Here's how the part is built. I have some questions about the finished solid (model axes, mm). A direction names the side the tool comes from. Give positions to 0.01 mm unless a question says otherwise; leave off trailing zeros. Loops run counter-clockwise (first coordinate to the right, second up) from the corner with the lowest first, then second, coordinate; pieces in that order, holes last.
Q1. Suppose I cut it at D-D (z = -16). List the corners of the cut face in (x, y) for me, and give its area (3 significant figures).
Q2. I need wall thicknesses on probe 1 along Z at (x, y) = (-2, 21); probe 2 along X at (y, z) = (17.75, -11.5); probe 3 along X at (y, z) = (29.2, -11.5) (3 decimals). Which ranges of each line are inside material? Lowest first, please.
Q3. Thinking about a two-plate mould opening in Y: for faces 1 (the face through (0, 30, -11)), 2 (the face through (2, 17, -20)), 3 (the face through (-2.5, 19, -1)), 4 (the face through (4.866, 28.521, -7.63)), which applies, pulls with the +Y half, pulls with the -Y half, needs draft (parallel to the pull), parting line crosses it, or undercut?
Q4. Suppose I cut it at B-B (z = -3.5). List the corners of the cut face in (x, y) for me (3 decimals), and give its area (3 significant figures).
Q5. Suppose I cut it at A-A (x = 2.5). Count the separate pieces of the cut face and the enclosed holes in it, and give its area (3 significant figures).
Q6. For faces 5 (the face through (3, 12, -1)), 6 (the face through (6, 15, -10)), 7 (the face through (4.55, 28.52, -4.24)), 8 (the face through (2, 1, -19)), 9 (the face through (-4, 10, -1)), which set-ups out of +Z, -Z, +X, -X, +Y, -Y let a thin tool reach every point of the face, with its end or its side?
```python
from build123d import *

# Parameters (mm, degrees)
EXTRUDE_1_DEPTH                  = 30
SKETCH_2_W                       = 4.5
SKETCH_2_H                       = 17
SKETCH_2_R                       = 1
EXTRUDE_2_DEPTH                  = 3
EXTRUDE_3_DEPTH                  = 27
PATTERN_LINEAR_1_COUNT           = 2
PATTERN_LINEAR_1_PITCH           = 5.5
PATTERN_LINEAR_2_COUNT           = 2
PATTERN_LINEAR_2_PITCH           = 5.5
CUT_EXTRUDE_1_REACH              = 39.108
SKETCH_5_W                       = 2.5
SKETCH_5_H                       = 3
PATTERN_LINEAR_3_COUNT           = 3
PATTERN_LINEAR_3_PITCH           = 7
PATTERN_LINEAR_4_COUNT           = 2
PATTERN_LINEAR_4_PITCH           = 5.5
PATTERN_LINEAR_4_COPY_1_REACH    = 39.108
PATTERN_LINEAR_4_COPY_1_SKETCH_W = 2.5
PATTERN_LINEAR_4_COPY_1_SKETCH_H = 3
PATTERN_LINEAR_4_COPY_2_REACH    = 39.108
PATTERN_LINEAR_4_COPY_2_SKETCH_W = 2.5
PATTERN_LINEAR_4_COPY_2_SKETCH_H = 3
CUT_EXTRUDE_2_REACH              = 39.108
SKETCH_6_W                       = 2.5
SKETCH_6_H                       = 5
PATTERN_LINEAR_5_COUNT           = 3
PATTERN_LINEAR_5_PITCH           = 7
PATTERN_LINEAR_7_COUNT           = 2
PATTERN_LINEAR_7_PITCH           = 5.5
PATTERN_LINEAR_7_COPY_1_REACH    = 39.108
PATTERN_LINEAR_7_COPY_1_SKETCH_W = 2.5
PATTERN_LINEAR_7_COPY_1_SKETCH_H = 5
PATTERN_LINEAR_7_COPY_2_REACH    = 39.108
PATTERN_LINEAR_7_COPY_2_SKETCH_W = 2.5
PATTERN_LINEAR_7_COPY_2_SKETCH_H = 5


with BuildPart() as part:
    # Эскиз1 → Бобышка-Вытянуть1 (new body)
    with BuildSketch(Plane(origin=(0, 0, 0), x_dir=(1, 0, 0), z_dir=(0, 1, 0))):
        Polygon((5, 0), (-5, 0), (-6, 1), (-6, 10.5), (-5, 10.5), (-5, 2), (-0.5, 2), (-0.5, 10.5), (0.5, 10.5), (0.5, 2), (5, 2), (5, 10.5), (6, 10.5), (6, 1), align=None)
    extrude_1 = extrude(amount=EXTRUDE_1_DEPTH)

    # Зеркальное отражение1: Бобышка-Вытянуть1 across plane
    add(extrude_1.mirror(Plane(origin=(-0.5, 30, -10.5), x_dir=(1, 0, 0), z_dir=(0, 0, 1))))

    # Эскиз2 → Бобышка-Вытянуть2 (add)
    with BuildSketch(Plane(origin=(0, 30, 0), x_dir=(1, 0, 0), z_dir=(0, 1, 0))):
        with Locations((-2.75, 10.5)):
            Rectangle(SKETCH_2_W, SKETCH_2_H)
        with Locations(Location((-1.625, 11.5, 0), (0, 0, 270))):
            Circle(SKETCH_2_R, mode=Mode.SUBTRACT)
        with Locations(Location((-1.625, 7.5, 0), (0, 0, 270))):
            Circle(SKETCH_2_R, mode=Mode.SUBTRACT)
        with Locations(Location((-1.625, 3.5, 0), (0, 0, 270))):
            Circle(SKETCH_2_R, mode=Mode.SUBTRACT)
    extrude_2 = extrude(amount=-EXTRUDE_2_DEPTH)

    # Эскиз3 → Бобышка-Вытянуть3 (add)
    with BuildSketch(Plane.XZ.offset(-27)):
        Polygon((-2.5, -19), (-0.5, -19), (-0.5, -13), (-1.625, -13), (-2.5, -13), align=None)
        Polygon((-1.625, -10), (-0.5, -10), (-0.5, -9), (-1.625, -9), (-2.5, -9), (-2.5, -10), align=None)
        Polygon((-1.625, -6), (-0.5, -6), (-0.5, -5), (-2.5, -5), (-2.5, -6), align=None)
    extrude_3 = extrude(amount=EXTRUDE_3_DEPTH)

    # Линейный массив1: Бобышка-Вытянуть2 ×2
    with Locations(*[(i * PATTERN_LINEAR_1_PITCH, 0, 0) for i in range(1, PATTERN_LINEAR_1_COUNT)]):
        add(extrude_2)

    # Линейный массив2: Бобышка-Вытянуть3 ×2
    with Locations(*[(i * PATTERN_LINEAR_2_PITCH, 0, 0) for i in range(1, PATTERN_LINEAR_2_COUNT)]):
        add(extrude_3)

    # Эскиз5 → Вырез-Вытянуть1 (cut, up to next)
    with BuildSketch(Plane(origin=(0, 0, -21), x_dir=(-1, 0, 0), z_dir=(0, 0, -1)), mode=Mode.PRIVATE) as cut_extrude_1_sk1:
        with Locations((3.75, 18.5)):
            Rectangle(SKETCH_5_W, SKETCH_5_H)
    cut_extrude_1_tool1 = extrude(cut_extrude_1_sk1.sketch, amount=-CUT_EXTRUDE_1_REACH, mode=Mode.PRIVATE) & part.part
    cut_extrude_1 = cut_extrude_1_tool1.solids().sort_by_distance((-3.75, 18.5, -21))[0]
    add(cut_extrude_1, mode=Mode.SUBTRACT)

    # Линейный массив3: Вырез-Вытянуть1 ×3
    with Locations(*[(0, -i * PATTERN_LINEAR_3_PITCH, 0) for i in range(1, PATTERN_LINEAR_3_COUNT)]):
        add(cut_extrude_1, mode=Mode.SUBTRACT)

    # Линейный массив4: Вырез-Вытянуть1 ×2
    with Locations(*[(i * PATTERN_LINEAR_4_PITCH, 0, 0) for i in range(1, PATTERN_LINEAR_4_COUNT)]):
        add(cut_extrude_1, mode=Mode.SUBTRACT)

    # Линейный массив4 copy 1 sketch → Линейный массив4 copy 1 (cut, up to next)
    with BuildSketch(Plane(origin=(5.5, -7, -21), x_dir=(-1, 0, 0), z_dir=(0, 0, -1)), mode=Mode.PRIVATE) as pattern_linear_4_copy_1_sk1:
        with Locations((3.75, 18.5)):
            Rectangle(PATTERN_LINEAR_4_COPY_1_SKETCH_W, PATTERN_LINEAR_4_COPY_1_SKETCH_H)
    pattern_linear_4_copy_1_tool1 = extrude(pattern_linear_4_copy_1_sk1.sketch, amount=-PATTERN_LINEAR_4_COPY_1_REACH, mode=Mode.PRIVATE) & part.part
    add(pattern_linear_4_copy_1_tool1.solids().sort_by_distance((1.75, 11.5, -21))[0], mode=Mode.SUBTRACT)

    # Линейный массив4 copy 2 sketch → Линейный массив4 copy 2 (cut, up to next)
    with BuildSketch(Plane(origin=(5.5, -14, -21), x_dir=(-1, 0, 0), z_dir=(0, 0, -1)), mode=Mode.PRIVATE) as pattern_linear_4_copy_2_sk1:
        with Locations((3.75, 18.5)):
            Rectangle(PATTERN_LINEAR_4_COPY_2_SKETCH_W, PATTERN_LINEAR_4_COPY_2_SKETCH_H)
    pattern_linear_4_copy_2_tool1 = extrude(pattern_linear_4_copy_2_sk1.sketch, amount=-PATTERN_LINEAR_4_COPY_2_REACH, mode=Mode.PRIVATE) & part.part
    add(pattern_linear_4_copy_2_tool1.solids().sort_by_distance((1.75, 4.5, -21))[0], mode=Mode.SUBTRACT)

    # Эскиз6 → Вырез-Вытянуть2 (cut, up to next)
    with BuildSketch(Plane.XY, mode=Mode.PRIVATE) as cut_extrude_2_sk1:
        with Locations((-3.75, 19.5)):
            Rectangle(SKETCH_6_W, SKETCH_6_H)
    cut_extrude_2_tool1 = extrude(cut_extrude_2_sk1.sketch, amount=-CUT_EXTRUDE_2_REACH, mode=Mode.PRIVATE) & part.part
    cut_extrude_2 = cut_extrude_2_tool1.solids().sort_by_distance((-3.75, 19.5, 0))[0]
    add(cut_extrude_2, mode=Mode.SUBTRACT)

    # Линейный массив5: Вырез-Вытянуть2 ×3
    with Locations(*[(0, -i * PATTERN_LINEAR_5_PITCH, 0) for i in range(1, PATTERN_LINEAR_5_COUNT)]):
        add(cut_extrude_2, mode=Mode.SUBTRACT)

    # Линейный массив7: Вырез-Вытянуть2 ×2
    with Locations(*[(i * PATTERN_LINEAR_7_PITCH, 0, 0) for i in range(1, PATTERN_LINEAR_7_COUNT)]):
        add(cut_extrude_2, mode=Mode.SUBTRACT)

    # Линейный массив7 copy 1 sketch → Линейный массив7 copy 1 (cut, up to next)
    with BuildSketch(Plane(origin=(5.5, -7, 0), x_dir=(1, 0, 0), z_dir=(0, 0, 1)), mode=Mode.PRIVATE) as pattern_linear_7_copy_1_sk1:
        with Locations((-3.75, 19.5)):
            Rectangle(PATTERN_LINEAR_7_COPY_1_SKETCH_W, PATTERN_LINEAR_7_COPY_1_SKETCH_H)
    pattern_linear_7_copy_1_tool1 = extrude(pattern_linear_7_copy_1_sk1.sketch, amount=-PATTERN_LINEAR_7_COPY_1_REACH, mode=Mode.PRIVATE) & part.part
    add(pattern_linear_7_copy_1_tool1.solids().sort_by_distance((1.75, 12.5, 0))[0], mode=Mode.SUBTRACT)

    # Линейный массив7 copy 2 sketch → Линейный массив7 copy 2 (cut, up to next)
    with BuildSketch(Plane(origin=(5.5, -14, 0), x_dir=(1, 0, 0), z_dir=(0, 0, 1)), mode=Mode.PRIVATE) as pattern_linear_7_copy_2_sk1:
        with Locations((-3.75, 19.5)):
            Rectangle(PATTERN_LINEAR_7_COPY_2_SKETCH_W, PATTERN_LINEAR_7_COPY_2_SKETCH_H)
    pattern_linear_7_copy_2_tool1 = extrude(pattern_linear_7_copy_2_sk1.sketch, amount=-PATTERN_LINEAR_7_COPY_2_REACH, mode=Mode.PRIVATE) & part.part
    add(pattern_linear_7_copy_2_tool1.solids().sort_by_distance((1.75, 5.5, 0))[0], mode=Mode.SUBTRACT)


solid = part.part
```
Solutions:
1. outline: (-6, 0) - (-5, 0) - (-5, 27) - (-2.5, 27) - (-2.5, 0) - (0.5, 0) - (0.5, 27) - (3, 27) - (3, 0) - (6, 0) - (6, 30) - (-6, 30) - close
1. area: 225 mm2
2. probe 1: z = -21 to -13, -10 to -9, -6 to -5, -2 to 0
2. probe 2: x = -6 to -5, -0.5 to 0.5, 5 to 6
2. probe 3: x = -6 to -2.625, -0.625 to 2.875, 4.875 to 6
3. face 1: pulls with the +Y half
3. face 2: undercut
3. face 3: undercut
3. face 4: needs draft
4. outline: (-6, 0) - (-5, 0) - (-5, 27) - (-2.625, 27) - (-2.625, 30) - (-6, 30) - close; (-0.625, 27) - (-0.5, 27) - (-0.5, 0) - (0.5, 0) - (0.5, 27) - (2.875, 27) - (2.875, 30) - (-0.625, 30) - close; (4.875, 27) - (5, 27) - (5, 0) - (6, 0) - (6, 30) - (4.875, 30) - close
4. area: 105 mm2
5. separate pieces: 7
5. enclosed holes: 0
5. area: 123 mm2
6. face 5: +Z
6. face 6: +Z, -Z, +X, +Y, -Y
6. face 7: +Y, -Y
6. face 8: -Y
6. face 9: +Z, -Z
